from build123d import *

# Parameters (mm, degrees)
CYLINDER001_R     = 8.8
CYLINDER001_DEPTH = 30
PAD_DEPTH         = 13
CHAMFER001_SIZE   = 1.5


with BuildPart() as cilindro001:
    # Cylinder001 → Cylinder001 (new body)
    with BuildSketch(Plane.XY.offset(-10)):
        Circle(CYLINDER001_R)
    extrude(amount=CYLINDER001_DEPTH)


with BuildPart() as revolution:
    # Sketch001 → Revolution (revolve)
    with BuildSketch(Plane.YZ):
        Polygon((23.594229, 8.5), (15.8, 13), (25.8, 13), (25.8, 0), (15.8, 0), (23.594229, 4.5), align=None)
    revolve(axis=Axis((0, 0, 0), (0, 0, 1)))


with BuildPart() as chamfer001:
    # Sketch → Pad (new body)
    with BuildSketch(Plane.XY):
        Polygon((9.237604, 16), (-9.237604, 16), (-18.475209, 0), (-9.237604, -16), (9.237604, -16), (18.475209, 0), align=None)
    extrude(amount=PAD_DEPTH)

    # Cut: cut Revolution
    add(revolution.part, mode=Mode.SUBTRACT)

    # Cut002: cut Cilindro001
    add(cilindro001.part, mode=Mode.SUBTRACT)

    # Chamfer001
    chamfer001_edges = [chamfer001.edges().sort_by_distance(p)[0] for p in [
        (-8.8, 0, 13),
        (-8.8, 0, 0),
    ]]
    chamfer(chamfer001_edges, length=CHAMFER001_SIZE)


solid = chamfer001.part
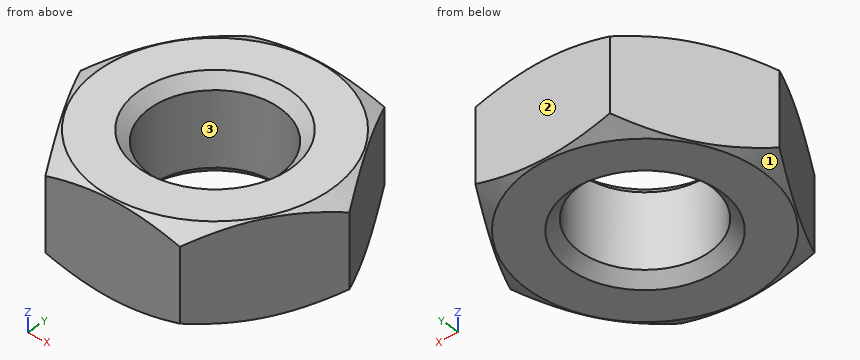
Source: CAD feature listing. Evaluate the final solid. Frame: model axes, mm. Face numbers are marked on the shaded views. Round coordinates to 2 decimals unless told otherwise and drop trailing zeros. Loops run counter-clockwise (first coordinate to the right, second up) from the corner with the lowest first, then second, coordinate; pieces in that order, holes last. Notation, with made-up numbers: M 33.5,32.5 L 84.5,32.5 A20 cw 84.5,46.5 Z; hole C 51.25,-16 d8. An arc over 180 degrees is marked long. Return JSON: item names as keys, results as strings. Group by question number.
1. Material intervals for line 1 along Y through (x, z) = (0, 6.5); line 2 along X through (y, z) = (0, 4.5); line 3 along Y through (x, z) = (-4, 9.25), sorted ascending. Write a range as from..to.
2. Pin query (flat end, axial travel): pin 1 (4 mm diameter, centred on y = -0.5, z = 3.5, fed in from +X); pin 2 (2 mm diameter, centred on x = -14.5, z = 5.5, fed in from +Y); pin 3 (5 mm diameter, centred on y = -6.5, z = 9, fed in from -X). Return the tip coordinate at first contact, or that it passes through.
3. Section query A-A on x = 0. Output: boundary loops of the cut face in (y, z), and give its area (3 significant figures).
4. Mould query, pull axis Y, two halves, no side actions, for the marked faces 1, 2 and 3. Classes: released by +Y, released by -Y, zero draft, split by the parting line, or undercut.
5. Section query B-B on z = 9. Output: boundary loops of the cut face in (x, y).
Checks:
{
 "1": {"line 1": "y = -16..-8.8, 8.8..16", "line 2": "x = -18.48..-8.8, 8.8..18.48", "line 3": "y = -16..-7.84, 7.84..16"},
 "2": {"pin 1": "stops at x = 18.48", "pin 2": "stops at y = 8.62", "pin 3": "stops at x = -16.17"},
 "3": {"outline": "M -16,0.12 L -15.8,0 L -10.3,0 L -8.8,1.5 L -8.8,11.5 L -10.3,13 L -15.8,13 L -16,12.88 Z; M 8.8,1.5 L 10.3,0 L 15.8,0 L 16,0.12 L 16,12.88 L 15.8,13 L 10.3,13 L 8.8,11.5 Z", "area": "183 mm²"},
 "4": {"face 1": "split by the parting line", "face 2": "released by +Y", "face 3": "undercut"},
 "5": {"outline": "M -18.48,0 L -9.24,-16 L 9.24,-16 L 18.48,0 L 9.24,16 L -9.24,16 Z; hole C 0,0 d17.6"}
}
